from build123d import *

# Parameters (mm, degrees)
SKETCH001_R = 2
SKETCH001_W = 4
SKETCH001_H = 13
PAD_DEPTH   = 2.8
FILLET_R    = 10
FILLET001_R = 10


with BuildPart() as part:
    # Sketch001 → Pad (new body)
    with BuildSketch(Plane.XY):
        with BuildLine():
            Line((48.718334, -1.052358), (47.718334, -1.052358))
            Line((47.718334, -1.052358), (47.718334, -14.052358))
            Line((47.718334, -14.052358), (48.718364, -14.052358))
            Line((48.718364, -14.052358), (48.718364, -57.149485))
            Line((-48.693828, -57.149485), (48.718364, -57.149485))
            Line((-48.693828, -57.149485), (-48.693828, -12.562763))
            Line((-48.693828, -12.562763), (-47.693828, -12.562763))
            Line((-47.693828, 0.437237), (-47.693828, -12.562763))
            Line((-48.693828, 0.437237), (-47.693828, 0.437237))
            Line((-48.693828, 0.437237), (-48.693828, 62.459473))
            ThreePointArc((48.718334, 60.727454), (0.866096, 109.615293), (-48.693828, 62.459473))
            Line((48.718334, -1.052358), (48.718334, 60.727454))
        make_face()
        with Locations((-16.731984, 74.31012)):
            Circle(SKETCH001_R, mode=Mode.SUBTRACT)
        with Locations((14.268016, 74.31012)):
            Circle(SKETCH001_R, mode=Mode.SUBTRACT)
        with Locations((-16.731984, 98.31012)):
            Circle(SKETCH001_R, mode=Mode.SUBTRACT)
        with Locations((14.268016, 98.31012)):
            Circle(SKETCH001_R, mode=Mode.SUBTRACT)
        with Locations((28.860233, -7.552358)):
            Rectangle(SKETCH001_W, SKETCH001_H, mode=Mode.SUBTRACT)
        with Locations((-28.454098, -6.062763)):
            Rectangle(SKETCH001_W, SKETCH001_H, mode=Mode.SUBTRACT)
        Polygon((7.593316, 9.361636), (7.593316, -4.638364), (5.519069, -4.638364), (5.519069, -5.138364), (-0.480931, -5.138364), (-0.480931, -4.638364), (-2.480931, -4.638364), (-2.480931, 9.361636), (-0.515563, 9.361636), (-0.515563, 9.861636), (5.484437, 9.861636), (5.484437, 9.361636), align=None, mode=Mode.SUBTRACT)
        Polygon((26.360233, -18.052358), (19.360233, -18.052358), (19.360233, -25.052358), (15.360233, -25.052358), (15.360233, -32.052358), (19.360233, -32.052358), (19.360233, -39.052358), (26.360233, -39.052358), (26.360233, -32.052358), (30.360233, -32.052358), (30.360233, -25.052358), (26.360233, -25.052358), align=None, mode=Mode.SUBTRACT)
        Polygon((-25.153265, -16.562763), (-25.153265, -23.562763), (-29.153265, -23.562763), (-29.153265, -30.562763), (-25.153265, -30.562763), (-25.153265, -37.562763), (-18.153265, -37.562763), (-18.153265, -30.562763), (-14.153265, -30.562763), (-14.153265, -23.562763), (-18.153265, -23.562763), (-18.153265, -16.562763), align=None, mode=Mode.SUBTRACT)
    extrude(amount=PAD_DEPTH)

    # Fillet
    fillet_edges = [part.edges().sort_by_distance(p)[0] for p in [
        (48.718364, -57.149485, 1.4),
    ]]
    fillet(fillet_edges, radius=FILLET_R)

    # Fillet001
    fillet001_edges = [part.edges().sort_by_distance(p)[0] for p in [
        (-48.693828, -57.149485, 1.4),
    ]]
    fillet(fillet001_edges, radius=FILLET001_R)


solid = part.part
Here's how the part is built. I have some questions about the finished solid (model axes, mm). Give positions to 0.01 mm unless a question says otherwise; leave off trailing zeros. Order: outer loops, then holes, each group sorted by start corner. A loop starts at its lowest first (then second) coordinate and runs counter-clockwise, first axis right, second up. Notation, with made-up numbers: M -15.75,22.5 L 29.25,22.5 A20 cw 29.25,61.5 Z; hole C 33.5,57.25 d4. An arc over 180 degrees is marked long. Answer as a JSON object with one key per item and string values. Group by question number.
1) Please list where these lines run through material, in increasing order: L1, parallel to X at y = 0, z = 2.6; L2, parallel to X at y = -32, z = 1.5; L3, parallel to Y at x = 13.5, z = 0.45. Write a range as [from, to].
2) We'd pull the mould along X, two halves only. Please class faces 1 (the cylindrical face through (-18.21, 75.66, 1.38)), 2 (the cylindrical face through (45.87, -54.14, 1.42)), 3 (the cylindrical face through (-17.17, 96.36, 1.38)), 4 (the flat face through (1, 27, 0)): pulls with the +X half, pulls with the -X half, needs draft (parallel to the pull), parting line crosses it, or undercut.
3) Suppose I cut it at B-B, the plane x = -21.5. Write out the boundary of the cut face in (y, z), plus the area to 3 significant figures.
4) Suppose I cut it at C-C, the plane z = 1.5. Count the separate pieces of the cut face and the enclosed holes in it, plus the area to 3 significant figures.
5) Suppose I cut it at D-D, the plane y = 94.5. Write out the boundary of the cut face in (x, z), plus the area to 3 significant figures.
6) I'm going to push flat-ended pins straight in: pin 1 Ø2 at (x, y) = (-11.5, 35.5) entering from -Z; pin 2 Ø3.5 at (x, y) = (-16.73, 74.31) entering from -Z; pin 3 Ø0.6 at (x, z) = (7, 2) entering from +Y; pin 4 Ø1 at (y, z) = (93, 1.5) entering from -X. Where does each tip first touch, or does it pass through?
7) Suppose I cut it at A-A, the plane y = 3.5. Write out the boundary of the cut face in (x, z), plus the area to 3 significant figures.
Results found:
{
 "1": {"L1": "[-47.69, -30.45], [-26.45, -2.48], [7.59, 48.72]", "L2": "[-48.69, -25.15], [-18.15, 15.36], [30.36, 48.72]", "L3": "[-57.15, 72.46], [76.16, 96.46], [100.16, 107.72]"},
 "2": {"face 1": "undercut", "face 2": "pulls with the +X half", "face 3": "undercut", "face 4": "needs draft"},
 "3": {"outline": "M -57.15,0 L -37.56,0 L -37.56,2.8 L -57.15,2.8 Z; M -16.56,0 L 104.62,0 L 104.62,2.8 L -16.56,2.8 Z", "area": "394 mm²"},
 "4": {"separate pieces": "1", "enclosed holes": "9", "area": "14,500 mm²"},
 "5": {"outline": "M -35.28,0 L 35.28,0 L 35.28,2.8 L -35.28,2.8 Z", "area": "198 mm²"},
 "6": {"pin 1": "z = 0", "pin 2": "through", "pin 3": "y = 109.16", "pin 4": "x = -37.08"},
 "7": {"outline": "M -48.69,0 L -2.48,0 L -2.48,2.8 L -48.69,2.8 Z; M 7.59,0 L 48.72,0 L 48.72,2.8 L 7.59,2.8 Z", "area": "245 mm²"}
}
